Design review of the part built by this model. Coordinates are the model's own, in mm. A direction names the side the tool comes from. Coordinates: 2 decimals unless noted, no trailing zeros. Write each loop counter-clockwise with the first axis right and the second up, starting at its lowest first coordinate (ties: lowest second). Pieces come first, ordered by that corner, then holes. Notation, with made-up numbers: M 11,-23 L 33,-23 A20 cw 33,6 Z; hole C 6,83.5 d8. An arc over 180 degrees is marked long. Write item = value, one per line.
```python
from build123d import *

# Parameters (mm, degrees)
SKETCH1_R           = 25.5
BOSS_EXTRUDE1_DEPTH = 11
SKETCH2_R           = 30
BOSS_EXTRUDE2_DEPTH = 7
SKETCH3_R           = 37.476082354
SKETCH3_R_2         = 24
CUT_EXTRUDE1_DEPTH  = 4.5
SKETCH5_R           = 6.5
CUT_EXTRUDE2_DEPTH  = 30.5


with BuildPart() as part:
    # Sketch1 → Boss-Extrude1 (new body)
    with BuildSketch(Plane.XY):
        Circle(SKETCH1_R)
    extrude(amount=BOSS_EXTRUDE1_DEPTH)

    # Sketch2 → Boss-Extrude2 (add)
    with BuildSketch(Plane(origin=(0, 0, 0), x_dir=(-1, 0, 0), z_dir=(0, 0, -1))):
        Circle(SKETCH2_R)
    extrude(amount=BOSS_EXTRUDE2_DEPTH)

    # Sketch3 → Cut-Extrude1 (cut)
    with BuildSketch(Plane.XY.offset(8)):
        Circle(SKETCH3_R)
        Circle(SKETCH3_R_2, mode=Mode.SUBTRACT)
    extrude(amount=-CUT_EXTRUDE1_DEPTH, mode=Mode.SUBTRACT)

    # Sketch5 → Cut-Extrude2 (cut)
    with BuildSketch(Plane(origin=(0, 0, -7), x_dir=(-1, 0, 0), z_dir=(0, 0, -1))):
        with Locations((0, 15)):
            Circle(SKETCH5_R)
        with Locations((-12.990381057, -7.5)):
            Circle(SKETCH5_R)
        with Locations((12.990381057, -7.5)):
            Circle(SKETCH5_R)
    extrude(amount=-CUT_EXTRUDE2_DEPTH, mode=Mode.SUBTRACT)


solid = part.part
```
Q1. Consider section C-C, the plane y = 0. State the section outline as (x, z) points.
Check result:
outline = M -30,-7 L 30,-7 L 30,0 L 25.5,0 L 25.5,3.5 L 24,3.5 L 24,8 L 25.5,8 L 25.5,11 L -25.5,11 L -25.5,8 L -24,8 L -24,3.5 L -25.5,3.5 L -25.5,0 L -30,0 Z
Q2. The part is to be moulded in two halves that separate along X. For faces 1 (the cylindrical face through (-5.5, -24.9, 1.7)), 2 (the flat face through (15, -19, 3.5)), 3 (the cylindrical face through (-7.832, -11.455, 1.874)), say which applies: +X half, -X half, draft (parallel to the pull), parting line (faces both ways), or undercut.
Check result:
face_1 = parting line
face_2 = draft
face_3 = undercut
Q3. For P1, Ø4, axis at y = -17.5, z = -1, coming from the -X side; P2, Ø1, axis at y = 17, z = -1, coming from the +X side; P3, Ø8, axis at x = -12.99, y = -7.5, coming from the -Z side; P4, Ø3, axis at x = -13.5, z = 7, coming from the +Y side, all flat-tipped, find the tip position at first contact; note any pin that passes through.
Check result:
P1 = -25.69
P2 = 25.05
P3 = through
P4 = 22.29
Q4. Consider section D-D, the plane y = -7.5. State the section outline as (x, z) points.
Check result:
outline = M -29.05,-7 L -19.49,-7 L -19.49,11 L -24.37,11 L -24.37,8 L -22.8,8 L -22.8,3.5 L -24.37,3.5 L -24.37,0 L -29.05,0 Z; M -6.49,-7 L 6.49,-7 L 6.49,11 L -6.49,11 Z; M 19.49,-7 L 29.05,-7 L 29.05,0 L 24.37,0 L 24.37,3.5 L 22.8,3.5 L 22.8,8 L 24.37,8 L 24.37,11 L 19.49,11 Z
Q5. Consider section A-A, the plane x = 0. State the section outline as (y, z) points.
Check result:
outline = M -30,-7 L 8.5,-7 L 8.5,11 L -25.5,11 L -25.5,8 L -24,8 L -24,3.5 L -25.5,3.5 L -25.5,0 L -30,0 Z; M 21.5,-7 L 30,-7 L 30,0 L 25.5,0 L 25.5,3.5 L 24,3.5 L 24,8 L 25.5,8 L 25.5,11 L 21.5,11 Z
Q6. Consider section B-B, the plane y = 15. State the section outline as (x, z) points (3 decimals), and give its area (3 significant figures).
Check result:
outline = M -25.981,-7 L -6.5,-7 L -6.5,11 L -20.622,11 L -20.622,8 L -18.735,8 L -18.735,3.5 L -20.622,3.5 L -20.622,0 L -25.981,0 Z; M 6.5,-7 L 25.981,-7 L 25.981,0 L 20.622,0 L 20.622,3.5 L 18.735,3.5 L 18.735,8 L 20.622,8 L 20.622,11 L 6.5,11 Z
area = 566 mm²
Q7. Wall thickness on line 1 (X direction, y = -3, z = -5.5); line 2 (Z direction, x = -23, y = 14); line 3 (X direction, y = -8.5, z = 10.25): over which ranges is each line inside the solid? List them lowest first.
Check result:
line_1 = -29.85 to -17.68, -8.3 to 8.3, 17.68 to 29.85
line_2 = -7 to 0
line_3 = -24.04 to -19.41, -6.57 to 6.57, 19.41 to 24.04
Q8. Machinability: for faces 4 (the cylindrical face through (-5.5, -24.9, 9.5)), 5 (the flat face through (0, 0, 11)), 6 (the cylindrical face through (-23.977, 1.055, 5.781)), which of the approach directions +Z, -Z, +X, -X, +Y, -Y give a long, thin tool a straight path to every point of the face, cutting with its end or side? Answer none if there is none.
Check result:
face_4 = +Z
face_5 = +Z, +X, -X, +Y, -Y
face_6 = none
